Model file for the job. Use its own axes, mm. Face numbers are marked on the shaded views. A direction names the side the tool comes from. Give positions to 0.01 mm unless a question says otherwise; leave off trailing zeros. Loops run counter-clockwise (first coordinate to the right, second up) from the corner with the lowest first, then second, coordinate; pieces in that order, holes last. Notation, with made-up numbers: (75.5, 51.25) - (134.5, 51.25) arc R16 cw to (134.5, 69.25) - close; hole circle Ø6 at (-28, -20). An arc over 180 degrees is marked (long way). Answer as CSV lines item,"result". Start each with the question number.
Item 1: Saw through at D-D on y = -48. Give the cut face in (x, z), plus the area to 3 significant figures.
Item 2: Saw through at A-A on z = 9.75. Give the cut face in (x, y), plus the area to 3 significant figures.
Item 3: Saw through at B-B on y = -27.5. Give the cut face in (x, z), plus the area to 3 significant figures.
Item 4: Pin check, flat tips, straight feed: pin 1 (3.5 mm diameter, centred on x = 3.5, y = -50, fed in from -Z); pin 2 (1.3 mm diameter, centred on x = 3, z = 3.5, fed in from +Y); pin 3 (2 mm diameter, centred on x = -2.5, y = -42.5, fed in from +Z); pin 4 (1.6 mm diameter, centred on x = -0.5, z = 24, fed in from +Y). Stop position of each tip, or through.
Item 5: Tool access for the marked faces 1 and 2: list every direction of +Z, -Z, +X, -X, +Y, -Y with a clear straight run to the whole face (end or side of a thin tool).
Item 6: Saw through at C-C on z = 6.5. Give the cut face in (x, y).
Item 7: Drill centre lines: L1, parallel to Y at x = -1, z = 16.25; L2, parallel to Y at x = 2, z = 5.5; L3, parallel to X at y = -11, z = 9.5. Where is each one in solid material? Low to high. Write a range as from..to.
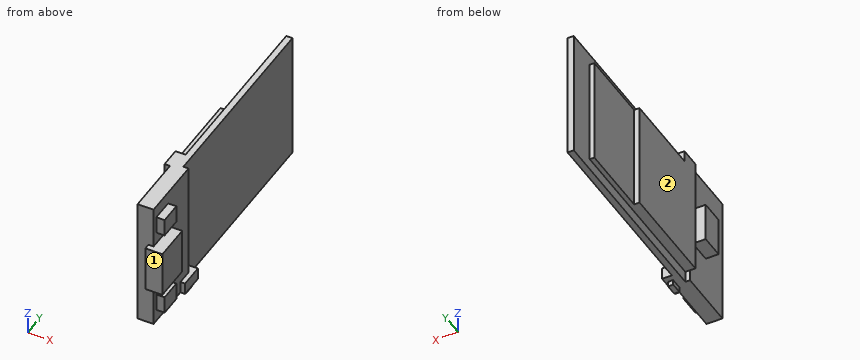
Autodesk Fusion 360 part; units mm, degrees
sketch "Sketch1" plane through (0, 0, 0) normal (1, 0, 0) x (0, 1, 0)
  line L0 (0, 0) -> (-51.5, 0)
  line L1 (-51.5, 0) -> (-51.5, 25.3)
  line L2 (-51.5, 25.3) -> (0, 25.3)
  line L3 (0, 25.3) -> (0, 0)
  dimension "d1" = 25.3
  dimension "d2" = 51.5
extrude "Extrude1" add sketch "Sketch1" along normal blind 1.2 makes body 1
sketch "Sketch2" plane through (0, -51.5, 0) normal (0, -1, 0) x (1, 0, 0)
  line L0 (0, 25.3) -> (0, 0)
  line L1 (0, 0) -> (1.2, 0)
  line L2 (1.2, 0) -> (1.2, 25.3)
  line L3 (1.2, 25.3) -> (0, 25.3)
  line L4 (1.2, 17.15) -> (4.5, 17.15)
  line L5 (4.5, 17.15) -> (4.5, 8.15)
  line L6 (4.5, 8.15) -> (1.2, 8.15)
  line L7 (1.2, 8.15) -> (1.2, 17.15)
  line L8 (4.5, 12.65) -> (1.2, 12.65)
  line L9 (1.2, 25.3) -> (1.2, 0)
  dimension "d5" = 9
  dimension "d7" = 4.5
extrude "Extrude2" add sketch "Sketch2" along normal blind 1.1 and the other way blind 6 separate body contours L2 L4 L5 L7 L8 L9 | L2 L5 L6 L7 L8 L9 makes body 2
sketch "Sketch3" plane through (1.2, 0, 0) normal (1, 0, 0) x (0, 1, 0)
  line L0 (0, 25.3) -> (-51.5, 25.3)
  line L1 (-51.5, 25.3) -> (-51.5, 0)
  line L2 (-51.5, 0) -> (0, 0)
  line L3 (0, 0) -> (0, 25.3)
  line L4 (-50.5, 22.9) -> (-46.3, 22.9)
  line L5 (-46.3, 22.9) -> (-46.3, 19.5)
  line L6 (-46.3, 19.5) -> (-50.5, 19.5)
  line L7 (-50.5, 19.5) -> (-50.5, 22.9)
  line L8 (0, 12.65) -> (-51.5, 12.65)
  line L9 (-46.3, 2.4) -> (-46.3, 5.8)
  line L10 (-50.5, 2.4) -> (-46.3, 2.4)
  line L11 (-50.5, 5.8) -> (-50.5, 2.4)
  line L12 (-46.3, 5.8) -> (-50.5, 5.8)
  dimension "d12" = 3.4
  dimension "d13" = 4.2
  dimension "d14" = 2.4
  dimension "d15" = 1
extrude "Extrude3" add sketch "Sketch3" along normal blind 2.6 contours L4 L5 L6 L7 | L9 L10 L11 L12 bodies 1
sketch "Sketch4" plane through (0, 0, 0) normal (-1, 0, 0) x (0, -1, 0)
  line L0 (51.5, 25.3) -> (0, 25.3)
  line L1 (0, 25.3) -> (0, 0)
  line L2 (0, 0) -> (51.5, 0)
  line L3 (51.5, 0) -> (51.5, 25.3)
  line L4 (40.9, 16.45) -> (45.5, 16.45)
  line L5 (45.5, 16.45) -> (45.5, 8.85)
  line L6 (45.5, 8.85) -> (40.9, 8.85)
  line L7 (40.9, 8.85) -> (40.9, 16.45)
  line L8 (51.5, 25.3) -> (51.5, 0)
  line L9 (40.9, 12.65) -> (45.5, 12.65)
  line L10 (51.5, 12.65) -> (0, 12.65)
  dimension "d18" = 7.6
  dimension "d19" = 4.6
  dimension "d20" = 6
extrude "Extrude4" add sketch "Sketch4" along normal blind 3.4 contours L4 L5 L7 L9 L10 | L5 L6 L7 L9 L10 bodies 1
sketch "Sketch5" plane through (1.2, 0, 0) normal (1, 0, 0) x (0, 1, 0)
  line L0 (-46.3, 5.8) -> (-46.3, 2.4)
  line L1 (-46.3, 2.4) -> (-50.5, 2.4)
  line L2 (-50.5, 2.4) -> (-50.5, 5.8)
  line L3 (-50.5, 5.8) -> (-46.3, 5.8)
  line L4 (-50.5, 19.5) -> (-50.5, 22.9)
  line L5 (-50.5, 22.9) -> (-46.3, 22.9)
  line L6 (-46.3, 22.9) -> (-46.3, 19.5)
  line L7 (-46.3, 19.5) -> (-50.5, 19.5)
  line L8 (0, 25.3) -> (-51.5, 25.3)
  line L9 (-51.5, 25.3) -> (-51.5, 0)
  line L10 (-51.5, 0) -> (0, 0)
  line L11 (0, 0) -> (0, 25.3)
  line L12 (-41.9, 0) -> (-37.3, 0)
  line L13 (-37.3, 0) -> (-37.3, 2.3)
  line L14 (-37.3, 2.3) -> (-41.9, 2.3)
  line L15 (-41.9, 2.3) -> (-41.9, 0)
  dimension "d23" = 4.6
  dimension "d24" = 2.3
  dimension "d25" = 14.2
extrude "Extrude5" add sketch "Sketch5" along normal blind 1.9 contours L10 L12 L13 L14 L15 bodies 1
sketch "Sketch6" plane through (0, 0, 0) normal (0, 0, -1) x (1, 0, 0)
  line L0 (0, 51.5) -> (0, 0)
  line L1 (0, 0) -> (1.2, 0)
  line L2 (1.2, 0) -> (1.2, 37.3)
  line L3 (1.2, 37.3) -> (3.1, 37.3)
  line L4 (3.1, 37.3) -> (3.1, 41.9)
  line L5 (3.1, 41.9) -> (1.2, 41.9)
  line L6 (1.2, 41.9) -> (1.2, 51.5)
  line L7 (1.2, 51.5) -> (0, 51.5)
  line L8 (1.6, 40.7) -> (2.6, 40.7)
  line L9 (2.6, 40.7) -> (2.6, 38.5)
  line L10 (2.6, 38.5) -> (1.6, 38.5)
  line L11 (1.6, 38.5) -> (1.6, 40.7)
  dimension "d28" = 1.2
  dimension "d29" = 1.2
  dimension "d30" = 0.5
  dimension "d31" = 1
extrude "Extrude6" add sketch "Sketch6" along normal blind 1 contours L8 L9 L10 L11 bodies 1
sketch "Sketch7" plane through (0, 0, 0) normal (-1, 0, 0) x (0, -1, 0)
  line L0 (40.9, 8.85) -> (40.9, 16.45)
  line L1 (40.9, 16.45) -> (45.5, 16.45)
  line L2 (45.5, 16.45) -> (45.5, 8.85)
  line L3 (45.5, 8.85) -> (40.9, 8.85)
  line L4 (51.5, 25.3) -> (0, 25.3)
  line L5 (0, 25.3) -> (0, 0)
  line L6 (0, 0) -> (51.5, 0)
  line L7 (51.5, 0) -> (51.5, 25.3)
  line L8 (39.9, 25.3) -> (19.9, 25.3)
  line L9 (19.9, 25.3) -> (19.9, 2.2)
  line L10 (19.9, 2.2) -> (39.9, 2.2)
  line L11 (39.9, 2.2) -> (39.9, 25.3)
  line L12 (39.9, 25.3) -> (51.5, 25.3)
  line L13 (51.5, 25.3) -> (51.5, 0)
  line L14 (51.5, 0) -> (39.9, 0)
  line L15 (39.9, 0) -> (39.9, 25.3)
  line L16 (5.7, 23.1) -> (19.9, 23.1)
  line L17 (19.9, 23.1) -> (19.9, 2.2)
  line L18 (19.9, 2.2) -> (5.7, 2.2)
  line L19 (5.7, 2.2) -> (5.7, 23.1)
  line L20 (19.9, 23.1) -> (36, 23.1)
  line L21 (36, 23.1) -> (36, 25.3)
  dimension "d34" = 1
  dimension "d35" = 20
  dimension "d36" = 2.2
  dimension "d37" = 5.7
  dimension "d38" = 2.2
  dimension "d39" = 2.2
  dimension "d40" = 36
extrude "Extrude7" add sketch "Sketch7" along normal blind 1.95 contours L4 L8 L9 L10 L11 L15 L17 L20 L21 bodies 1
extrude "Extrude8" add sketch "Sketch7" along normal blind 0.9 contours L4 L6 L7 L11 L12 L13 L14 L15 | L9 L16 L17 L18 L19 bodies 1
sketch "Sketch8" plane through (1.2, 0, 0) normal (1, 0, 0) x (0, 1, 0)
  line L0 (-37.3, 2.3) -> (-37.3, 0)
  line L1 (-37.3, 0) -> (0, 0)
  line L2 (0, 0) -> (0, 25.3)
  line L3 (0, 25.3) -> (-51.5, 25.3)
  line L4 (-51.5, 25.3) -> (-51.5, 0)
  line L5 (-51.5, 0) -> (-41.9, 0)
  line L6 (-41.9, 0) -> (-41.9, 2.3)
  line L7 (-41.9, 2.3) -> (-37.3, 2.3)
  line L8 (-46.3, 5.8) -> (-46.3, 2.4)
  line L9 (-46.3, 2.4) -> (-50.5, 2.4)
  line L10 (-50.5, 2.4) -> (-50.5, 5.8)
  line L11 (-50.5, 5.8) -> (-46.3, 5.8)
  line L12 (-50.5, 19.5) -> (-50.5, 22.9)
  line L13 (-50.5, 22.9) -> (-46.3, 22.9)
  line L14 (-46.3, 22.9) -> (-46.3, 19.5)
  line L15 (-46.3, 19.5) -> (-50.5, 19.5)
  line L16 (-51.5, 25.3) -> (-39, 25.3)
  line L17 (-39, 25.3) -> (-39, 0)
  line L18 (-39, 0) -> (-51.5, 0)
  line L19 (-51.5, 0) -> (-51.5, 25.3)
  dimension "d45" = 12.5
extrude "Extrude9" add sketch "Sketch8" along normal blind 1 contours L3 L4 L5 L6 L7 L16 L17 L18 L19 bodies 2 1
equation "d38 = d36"
equation "d39 = d38"
equation "d41 = 3.15 mm - 1.2 mm"
equation "d43 = 2.1 mm - 1.2 mm"
Responses:
1,outline,"(-0.9, 0) - (2.2, 0) - (2.2, 2.4) - (3.8, 2.4) - (3.8, 5.8) - (2.2, 5.8) - (2.2, 8.15) - (4.5, 8.15) - (4.5, 17.15) - (2.2, 17.15) - (2.2, 19.5) - (3.8, 19.5) - (3.8, 22.9) - (2.2, 22.9) - (2.2, 25.3) - (-0.9, 25.3) - close"
1,area,"110 mm2"
2,outline,"(-3.4, -45.5) - (-0.9, -45.5) - (-0.9, -51.5) - (1.2, -51.5) - (1.2, -52.6) - (4.5, -52.6) - (4.5, -45.5) - (2.2, -45.5) - (2.2, -39) - (1.2, -39) - (1.2, 0) - (0, 0) - (0, -5.7) - (-0.9, -5.7) - (-0.9, -19.9) - (-1.95, -19.9) - (-1.95, -39.9) - (-0.9, -39.9) - (-0.9, -40.9) - (-3.4, -40.9) - close"
2,area,"165 mm2"
3,outline,"(-1.95, 2.2) - (0, 2.2) - (0, 0) - (1.2, 0) - (1.2, 25.3) - (0, 25.3) - (0, 23.1) - (-1.95, 23.1) - close"
3,area,"71.1 mm2"
4,pin 1,"z = 0"
4,pin 2,"y = -46.3"
4,pin 3,"z = 16.45"
4,pin 4,"y = 0"
5,face 1,"+Z, -Z, +X, -X, -Y"
5,face 2,"+Z, -Z, -X, +Y"
6,outline,"(-1.95, -39.9) - (-0.9, -39.9) - (-0.9, -51.5) - (2.2, -51.5) - (2.2, -39) - (1.2, -39) - (1.2, 0) - (0, 0) - (0, -5.7) - (-0.9, -5.7) - (-0.9, -19.9) - (-1.95, -19.9) - close"
7,L1,"-45.5..-40.9, -39.9..-19.9"
7,L2,"-51.5..-39"
7,L3,"-0.9..1.2"
